Read the model definition and answer for the solid it produces. Units are mm, in the model's axes. A direction names the side the tool comes from. Give positions to 0.01 mm unless a question says otherwise; leave off trailing zeros. Order: outer loops, then holes, each group sorted by start corner. A loop starts at its lowest first (then second) coordinate and runs counter-clockwise, first axis right, second up. Notation, with made-up numbers: (58, 84) - (89, 84) arc R21 cw to (89, 113) - close; hole circle Ø3 at (73.5, 80.5). An arc over 180 degrees is marked (long way). Write each question's results on one line, items separated by ' | '.
from build123d import *

# Parameters (mm, degrees)
SKETCH1_W           = 120
SKETCH1_H           = 70
BOSS_EXTRUDE1_DEPTH = 2
SKETCH6_R           = 2
BOSS_EXTRUDE2_DEPTH = 11
SKETCH4_R           = 3.25
CUT_EXTRUDE2_DEPTH  = 11
SKETCH3_R           = 4.25
BOSS_EXTRUDE3_DEPTH = 6
SKETCH8_R           = 1.75
CUT_EXTRUDE6_DEPTH  = 8
SKETCH9_R           = 3.25
CUT_EXTRUDE8_DEPTH  = 4


with BuildPart() as part:
    # Sketch1 → Boss-Extrude1 (new body)
    with BuildSketch(Plane(origin=(0, 0, 0), x_dir=(1, 0, 0), z_dir=(0, 1, 0))):
        Rectangle(SKETCH1_W, SKETCH1_H)
    extrude(amount=BOSS_EXTRUDE1_DEPTH)

    # Sketch6 → Boss-Extrude2 (add)
    with BuildSketch(Plane(origin=(0, 2, 0), x_dir=(1, 0, 0), z_dir=(0, 1, 0))):
        with Locations(Location((0, -13, 0), (0, 0, 270))):
            Circle(SKETCH6_R)
        with Locations(Location((0, 13, 0), (0, 0, 270))):
            Circle(SKETCH6_R)
    extrude(amount=-BOSS_EXTRUDE2_DEPTH)

    # Sketch4 → Cut-Extrude2 (cut)
    with BuildSketch(Plane(origin=(0, 2, 0), x_dir=(1, 0, 0), z_dir=(0, 1, 0))):
        with Locations(Location((-27.054448087, -13.122273409, 0), (0, 0, 270))):
            Circle(SKETCH4_R)
        with Locations(Location((-27.023483048, -0.10764713, 0), (0, 0, 270))):
            Circle(SKETCH4_R)
        with Locations(Location((-27.081562274, 12.864019897, 0), (0, 0, 270))):
            Circle(SKETCH4_R)
        with Locations(Location((-13.567081484, 0, 0), (0, 0, 270))):
            Circle(SKETCH4_R)
        with Locations(Location((-13.567081484, -13, 0), (0, 0, 270))):
            Circle(SKETCH4_R)
        with Locations(Location((-13.567081484, 13, 0), (0, 0, 270))):
            Circle(SKETCH4_R)
        with Locations(Location((0, 0, 0), (0, 0, 270))):
            Circle(SKETCH4_R)
    extrude(amount=-CUT_EXTRUDE2_DEPTH, mode=Mode.SUBTRACT)

    # Sketch3 → Boss-Extrude3 (add)
    with BuildSketch(Plane(origin=(0, 2, 0), x_dir=(1, 0, 0), z_dir=(0, 1, 0))):
        with Locations(Location((-53.5, 28.5, 0), (0, 0, 270))):
            Circle(SKETCH3_R)
        with Locations(Location((53.5, 28.5, 0), (0, 0, 270))):
            Circle(SKETCH3_R)
        with Locations(Location((-53.5, -28.5, 0), (0, 0, 270))):
            Circle(SKETCH3_R)
        with Locations(Location((53.5, -28.5, 0), (0, 0, 270))):
            Circle(SKETCH3_R)
    extrude(amount=-BOSS_EXTRUDE3_DEPTH)

    # Sketch8 → Cut-Extrude6 (cut)
    with BuildSketch(Plane(origin=(0, 2, 0), x_dir=(1, 0, 0), z_dir=(0, 1, 0))):
        with Locations(Location((-53.5, 28.5, 0), (0, 0, 270))):
            Circle(SKETCH8_R)
        with Locations(Location((-53.5, -28.5, 0), (0, 0, 270))):
            Circle(SKETCH8_R)
        with Locations(Location((53.5, -28.5, 0), (0, 0, 270))):
            Circle(SKETCH8_R)
        with Locations(Location((53.5, 28.5, 0), (0, 0, 270))):
            Circle(SKETCH8_R)
    extrude(amount=-CUT_EXTRUDE6_DEPTH, mode=Mode.SUBTRACT)

    # Sketch9 → Cut-Extrude8 (cut)
    with BuildSketch(Plane(origin=(0, 2, 0), x_dir=(1, 0, 0), z_dir=(0, 1, 0))):
        with Locations(Location((-53.5, 28.5, 0), (0, 0, 270))):
            Circle(SKETCH9_R)
        with Locations(Location((53.5, 28.5, 0), (0, 0, 270))):
            Circle(SKETCH9_R)
        with Locations(Location((-53.5, -28.5, 0), (0, 0, 270))):
            Circle(SKETCH9_R)
        with Locations(Location((53.5, -28.5, 0), (0, 0, 270))):
            Circle(SKETCH9_R)
    extrude(amount=-CUT_EXTRUDE8_DEPTH, mode=Mode.SUBTRACT)


solid = part.part
(1) Each of these flat-tipped pins is pushed along its axis until it touches: pin 1 (4 mm diameter, centred on x = -39, z = 5, fed in from -Y); pin 2 (3 mm diameter, centred on x = -52.5, z = -29.5, fed in from +Y); pin 3 (7 mm diameter, centred on x = 54, z = -27, fed in from -Y). Where does it stop, or does it pass through?
Conclusion:
pin 1: y = 0 | pin 2: y = -2 | pin 3: y = -4
(2) Section B-B (z = -28.5) is taken. Give the vertices of the cut face in (x, y), plus the area to 3 significant figures.
Conclusion:
outline: (-60, 0) - (-57.75, 0) - (-57.75, -4) - (-55.25, -4) - (-55.25, -2) - (-56.75, -2) - (-56.75, 2) - (-60, 2) - close; (-51.75, -4) - (-49.25, -4) - (-49.25, 0) - (49.25, 0) - (49.25, -4) - (51.75, -4) - (51.75, -2) - (50.25, -2) - (50.25, 2) - (-50.25, 2) - (-50.25, -2) - (-51.75, -2) - close; (55.25, -4) - (57.75, -4) - (57.75, 0) - (60, 0) - (60, 2) - (56.75, 2) - (56.75, -2) - (55.25, -2) - close | area: 242 mm^2
(3) Section D-D (y = -7.75) is taken. Give the vertices of the cut face in (x, z), plus the area to 3 significant figures.
Conclusion:
outline: circle Ø4 at (0, -13); circle Ø4 at (0, 13) | area: 25.1 mm^2
(4) For faces 1 (the face through (-1.2, -4.4, 11.4)), 2 (the face through (-10.345, 1.014, -0.423)), 3 (the face through (-55, -2, 30)), determine the directions among +Z, -Z, +X, -X, +Y, -Y from which every point of the face is accessible in a straight line to the end or side of a thin tool.
Conclusion:
face 1: -Y | face 2: +Y, -Y | face 3: +Y
(5) Section C-C (x = 0) is taken. Give the vertices of the cut face in (y, z), plus the area to 3 significant figures.
Conclusion:
outline: (-9, -15) - (0, -15) - (0, -35) - (2, -35) - (2, -3.25) - (0, -3.25) - (0, -11) - (-9, -11) - close; (-9, 11) - (0, 11) - (0, 3.25) - (2, 3.25) - (2, 35) - (0, 35) - (0, 15) - (-9, 15) - close | area: 199 mm^2
(6) Consider probe 1 along X at (y, z) = (1.55, 0); probe 2 along X at (y, z) = (1, -28.5); probe 3 along X at (y, z) = (-1.1, 28.5). Determine where each line is inside the solid, lowest interval first. Write a range as [from, to].
Conclusion:
probe 1: [-60, -30.27], [-23.78, -16.82], [-10.32, -3.25], [3.25, 60] | probe 2: [-60, -56.75], [-50.25, 50.25], [56.75, 60] | probe 3: [-57.75, -56.75], [-50.25, -49.25], [49.25, 50.25], [56.75, 57.75]
(7) Section A-A (x = 53.5) is taken. Give the vertices of the cut face in (y, z), plus the area to 3 significant figures.
Conclusion:
outline: (-4, -32.75) - (0, -32.75) - (0, -35) - (2, -35) - (2, -31.75) - (-2, -31.75) - (-2, -30.25) - (-4, -30.25) - close; (-4, -26.75) - (-2, -26.75) - (-2, -25.25) - (2, -25.25) - (2, 25.25) - (-2, 25.25) - (-2, 26.75) - (-4, 26.75) - (-4, 24.25) - (0, 24.25) - (0, -24.25) - (-4, -24.25) - close; (-4, 30.25) - (-2, 30.25) - (-2, 31.75) - (2, 31.75) - (2, 35) - (0, 35) - (0, 32.75) - (-4, 32.75) - close | area: 142 mm^2
(8) The mould has two halves that part along Z. Classify faces 4 (the face through (-54.4, -4, -26.7)), 5 (the face through (50.617, 0.028, 30)), 6 (the face through (-55, -2, -27)): pulls with the +Z half, pulls with the -Z half, needs draft (parallel to the pull), parting line crosses it, or undercut.
Conclusion:
face 4: needs draft | face 5: undercut | face 6: undercut
